Check sheet for the modelled part. Datum: model origin and axes. Units: mm. A direction names the side the tool comes from. Round coordinates to 2 decimals unless told otherwise and drop trailing zeros. Write each loop counter-clockwise with the first axis right and the second up, starting at its lowest first coordinate (ties: lowest second). Pieces come first, ordered by that corner, then holes.
from build123d import *

# Parameters (mm, degrees)
SKETCH1_W             = 25.4
SKETCH1_H             = 25.4
BOSS_EXTRUDE1_DEPTH   = 1231.9
BOSS_EXTRUDE1_2_DEPTH = 1231.9
BOSS_EXTRUDE1_3_DEPTH = 1231.9
BOSS_EXTRUDE1_4_DEPTH = 1231.9
SKETCH2_W             = 25.4
SKETCH2_H             = 25.4
BOSS_EXTRUDE2_DEPTH   = 596.9
SKETCH3_W             = 25.4
SKETCH3_H             = 25.4
BOSS_EXTRUDE3_DEPTH   = 406.4
SKETCH4_W             = 25.4
SKETCH4_H             = 25.4
BOSS_EXTRUDE4_DEPTH   = 406.4
BOSS_EXTRUDE5_REACH   = 1445.225
SKETCH5_W             = 25.4
SKETCH5_H             = 25.4


with BuildPart() as part:
    # Sketch1 → Boss-Extrude1 (new body)
    with BuildSketch(Plane(origin=(0, 0, 0), x_dir=(1, 0, 0), z_dir=(0, 1, 0))):
        with Locations((-12.7, 12.7)):
            Rectangle(SKETCH1_W, SKETCH1_H)
    extrude(amount=BOSS_EXTRUDE1_DEPTH)



with BuildPart() as body_2:
    # Sketch1 → Boss-Extrude1 2 (new body)
    with BuildSketch(Plane(origin=(0, 0, 0), x_dir=(1, 0, 0), z_dir=(0, 1, 0))):
        with Locations((-12.7, 444.5)):
            Rectangle(SKETCH1_W, SKETCH1_H)
    extrude(amount=BOSS_EXTRUDE1_2_DEPTH)


with BuildPart() as body_3:
    # Sketch1 → Boss-Extrude1 3 (new body)
    with BuildSketch(Plane(origin=(0, 0, 0), x_dir=(1, 0, 0), z_dir=(0, 1, 0))):
        with Locations((241.3, 12.7)):
            Rectangle(SKETCH1_W, SKETCH1_H)
    extrude(amount=BOSS_EXTRUDE1_3_DEPTH)


with BuildPart() as body_4:
    # Sketch1 → Boss-Extrude1 4 (new body)
    with BuildSketch(Plane(origin=(0, 0, 0), x_dir=(1, 0, 0), z_dir=(0, 1, 0))):
        with Locations((241.3, 444.5)):
            Rectangle(SKETCH1_W, SKETCH1_H)
    extrude(amount=BOSS_EXTRUDE1_4_DEPTH)


with BuildPart() as part_1:
    add(part.part)

    add(body_2.part)  # Boss-Extrude2 merges body 2

    add(body_3.part)  # Boss-Extrude2 merges body 3

    add(body_4.part)  # Boss-Extrude2 merges body 4
    # Sketch2 → Boss-Extrude2 (add)
    with BuildSketch(Plane(origin=(0, 0, 0), x_dir=(0, 0, -1), z_dir=(1, 0, 0))):
        with Locations((12.7, 12.7)):
            Rectangle(SKETCH2_W, SKETCH2_H)
        with Locations((444.5, 12.7)):
            Rectangle(SKETCH2_W, SKETCH2_H)
        with Locations((228.6, 12.7)):
            Rectangle(SKETCH2_W, SKETCH2_H)
    extrude(amount=BOSS_EXTRUDE2_DEPTH)

    # Sketch3 → Boss-Extrude3 (add)
    with BuildSketch(Plane(origin=(0, 0, -25.4), x_dir=(-1, 0, 0), z_dir=(0, 0, -1))):
        with Locations((12.7, 12.7)):
            Rectangle(SKETCH3_W, SKETCH3_H)
        with Locations((-584.2, 12.7)):
            Rectangle(SKETCH3_W, SKETCH3_H)
    extrude(amount=BOSS_EXTRUDE3_DEPTH)

    # Sketch4 → Boss-Extrude4 (add)
    with BuildSketch(Plane.XY.offset(-431.8)):
        with Locations((241.3, 12.7)):
            Rectangle(SKETCH4_W, SKETCH4_H)
        with Locations((241.3, 1219.2)):
            Rectangle(SKETCH4_W, SKETCH4_H)
        with Locations((-12.7, 1219.2)):
            Rectangle(SKETCH4_W, SKETCH4_H)
        with Locations((241.3, 749.3)):
            Rectangle(SKETCH4_W, SKETCH4_H)
        with Locations((-12.7, 749.3)):
            Rectangle(SKETCH4_W, SKETCH4_H)
    extrude(amount=BOSS_EXTRUDE4_DEPTH)

    # Sketch5 → Boss-Extrude5 (add, up to next)
    with BuildSketch(Plane(origin=(0, 0, 0), x_dir=(0, 0, -1), z_dir=(1, 0, 0)), mode=Mode.PRIVATE) as boss_extrude5_sk1:
        with Locations((12.7, 1219.2)):
            Rectangle(SKETCH5_W, SKETCH5_H)
    boss_extrude5_tool1 = extrude(boss_extrude5_sk1.sketch, amount=BOSS_EXTRUDE5_REACH, mode=Mode.PRIVATE) - part_1.part
    # Sketch5 → Boss-Extrude5 (add, up to next)
    with BuildSketch(Plane(origin=(0, 0, 0), x_dir=(0, 0, -1), z_dir=(1, 0, 0)), mode=Mode.PRIVATE) as boss_extrude5_sk2:
        with Locations((444.5, 1219.2)):
            Rectangle(SKETCH5_W, SKETCH5_H)
    boss_extrude5_tool2 = extrude(boss_extrude5_sk2.sketch, amount=BOSS_EXTRUDE5_REACH, mode=Mode.PRIVATE) - part_1.part
    # Sketch5 → Boss-Extrude5 (add, up to next)
    with BuildSketch(Plane(origin=(0, 0, 0), x_dir=(0, 0, -1), z_dir=(1, 0, 0)), mode=Mode.PRIVATE) as boss_extrude5_sk3:
        with Locations((444.5, 749.3)):
            Rectangle(SKETCH5_W, SKETCH5_H)
    boss_extrude5_tool3 = extrude(boss_extrude5_sk3.sketch, amount=BOSS_EXTRUDE5_REACH, mode=Mode.PRIVATE) - part_1.part
    # Sketch5 → Boss-Extrude5 (add, up to next)
    with BuildSketch(Plane(origin=(0, 0, 0), x_dir=(0, 0, -1), z_dir=(1, 0, 0)), mode=Mode.PRIVATE) as boss_extrude5_sk4:
        with Locations((12.7, 749.3)):
            Rectangle(SKETCH5_W, SKETCH5_H)
    boss_extrude5_tool4 = extrude(boss_extrude5_sk4.sketch, amount=BOSS_EXTRUDE5_REACH, mode=Mode.PRIVATE) - part_1.part
    add(boss_extrude5_tool1.solids().sort_by_distance((0, 1219.2, -12.7))[0])
    add(boss_extrude5_tool2.solids().sort_by_distance((0, 1219.2, -444.5))[0])
    add(boss_extrude5_tool3.solids().sort_by_distance((0, 749.3, -444.5))[0])
    add(boss_extrude5_tool4.solids().sort_by_distance((0, 749.3, -12.7))[0])


solid = part_1.part
1. Release check for a two-part mould opening along Z. For faces 1 (the flat face through (238, 476, -457.2)), 2 (the flat face through (228.6, 376, -13)), 3 (the flat face through (228.6, 1219, -226)), 4 (the flat face through (-13, 376, -431.8)) record: released by +Z, released by -Z, zero draft, split by the parting line, or undercut.
2. Sectioned sample at B-B, the plane y = 778.5. Enter the section's corners in (x, z).
3. Scan line: line 1 along Y through (x, z) = (277, -237). Record every from-to range of solid material in increasing order.
4. Set-up check for faces 5 (the flat face through (113, 1219, -25.4)), 6 (the flat face through (113, 762, -444)), 7 (the flat face through (238, 0, -213)), 8 (the flat face through (241, 376, -25.4)): record each of +Z, -Z, +X, -X, +Y, -Y from which the full face is reachable in a straight line by a thin tool's end or side.
5. Sectioned sample at C-C, the plane z = -145. Enter the section's corners in (x, y), plus the area to 3 significant figures.
6. Sectioned sample at A-A, the plane z = -228. Enter the section's corners in (x, y).
7. Go/stop test with a flat-tipped pin: pin 1 (7.5 mm diameter, centred on y = 307.5, z = -14, fed in from +X). Record where the tip stops, or that it passes through.
8. Sectioned sample at D-D, the plane x = 332. Enter the section's corners in (y, z).
Computed values:
1. face 1: released by -Z
1. face 2: zero draft
1. face 3: undercut
1. face 4: undercut
2. outline: (-25.4, -457.2) - (0, -457.2) - (0, -431.8) - (-25.4, -431.8) - close; (-25.4, -25.4) - (0, -25.4) - (0, 0) - (-25.4, 0) - close; (228.6, -457.2) - (254, -457.2) - (254, -431.8) - (228.6, -431.8) - close; (228.6, -25.4) - (254, -25.4) - (254, 0) - (228.6, 0) - close
3. line 1: y = 0 to 25.4
4. face 5: +Y, -Y
4. face 6: +Z, -Z
4. face 7: +Z, -Z, +X, -X, -Y
4. face 8: +X, -X
5. outline: (-25.4, 0) - (0, 0) - (0, 25.4) - (-25.4, 25.4) - close; (-25.4, 736.6) - (0, 736.6) - (0, 762) - (-25.4, 762) - close; (-25.4, 1206.5) - (0, 1206.5) - (0, 1231.9) - (-25.4, 1231.9) - close; (228.6, 0) - (254, 0) - (254, 25.4) - (228.6, 25.4) - close; (228.6, 736.6) - (254, 736.6) - (254, 762) - (228.6, 762) - close; (228.6, 1206.5) - (254, 1206.5) - (254, 1231.9) - (228.6, 1231.9) - close; (571.5, 0) - (596.9, 0) - (596.9, 25.4) - (571.5, 25.4) - close
5. area: 4,520 mm2
6. outline: (-25.4, 0) - (596.9, 0) - (596.9, 25.4) - (-25.4, 25.4) - close; (-25.4, 736.6) - (0, 736.6) - (0, 762) - (-25.4, 762) - close; (-25.4, 1206.5) - (0, 1206.5) - (0, 1231.9) - (-25.4, 1231.9) - close; (228.6, 736.6) - (254, 736.6) - (254, 762) - (228.6, 762) - close; (228.6, 1206.5) - (254, 1206.5) - (254, 1231.9) - (228.6, 1231.9) - close
7. pin 1: stops at x = 254
8. outline: (0, -457.2) - (25.4, -457.2) - (25.4, -431.8) - (0, -431.8) - close; (0, -241.3) - (25.4, -241.3) - (25.4, -215.9) - (0, -215.9) - close; (0, -25.4) - (25.4, -25.4) - (25.4, 0) - (0, 0) - close
